from build123d import *

# Parameters (mm, degrees)
F0_W     = 38
F0_H     = 38
F0_R     = 2.25
F0_R_2   = 3.5
F1_DEPTH = 4
F2_DEPTH = 1
F3_DEPTH = 6
F4_R     = 5


with BuildPart() as f1:
    # F0 (on Top) → F1 (new body)
    with BuildSketch(Plane.XY):
        Rectangle(F0_W, F0_H)
        with Locations((-13, -13)):
            Circle(F0_R, mode=Mode.SUBTRACT)
        with Locations((13, -13)):
            Circle(F0_R, mode=Mode.SUBTRACT)
        with Locations((-13, 13)):
            Circle(F0_R, mode=Mode.SUBTRACT)
        Circle(F0_R_2, mode=Mode.SUBTRACT)
        with Locations((13, 13)):
            Circle(F0_R, mode=Mode.SUBTRACT)
        Circle(F0_R_2)
        Circle(F0_R, mode=Mode.SUBTRACT)
        Circle(F0_R)
    extrude(amount=-F1_DEPTH)

    # F0 (on Top) → F2 (join)
    with BuildSketch(Plane.XY):
        Circle(F0_R_2)
        Circle(F0_R, mode=Mode.SUBTRACT)
    extrude(amount=F2_DEPTH)

    # F0 (on Top) → F3 (join)
    with BuildSketch(Plane.XY):
        Circle(F0_R)
    extrude(amount=F3_DEPTH)

    # F4
    f4_edges = [f1.edges().sort_by_distance(p)[0] for p in [
        (-19, -19, -2),
        (19, -19, -2),
        (19, 19, -2),
        (-19, 19, -2),
    ]]
    fillet(f4_edges, radius=F4_R)


solid = f1.part
Input: part model. Units: mm. Frame: model coordinates. A direction names the side the tool comes from. Coordinates: 2 decimals unless noted, no trailing zeros. Order: outer loops, then holes, each group sorted by start corner. A loop starts at its lowest first (then second) coordinate and runs counter-clockwise, first axis right, second up.
1. Cut plane D-D, the plane y = 0. Return loops of the section in (x, z).
Checked values:
outline: (-19, -4) - (19, -4) - (19, 0) - (3.5, 0) - (3.5, 1) - (2.25, 1) - (2.25, 6) - (-2.25, 6) - (-2.25, 1) - (-3.5, 1) - (-3.5, 0) - (-19, 0) - close
2. Ray query, line 1 along Y through (x, z) = (13, -1.7); line 2 along Z through (x, y) = (8.5, 16.5); line 3 along X through (y, z) = (2, 3.5). Return the intervals inside material, ascending.
Checked values:
line 1: y = -19 to -15.25, -10.75 to 10.75, 15.25 to 19
line 2: z = -4 to 0
line 3: x = -1.03 to 1.03
3. Access query for faces 1 (the flat face through (0.7, -2.3, 1)), 2 (the flat face through (0, -19, -2)). Directions: +Z, -Z, +X, -X, +Y, -Y. A direction counts if a zero-diameter tool reaches every point of the face in a straight line with its end or side. Return the directions, or none.
Checked values:
face 1: +Z
face 2: +Z, -Z, +X, -X, -Y
4. Cut plane C-C, the plane z = -3.25. Return loops of the section in (x, y), plus the area to 3 significant figures.
Checked values:
outline: (-19, -14) arc R5 ccw to (-14, -19) - (14, -19) arc R5 ccw to (19, -14) - (19, 14) arc R5 ccw to (14, 19) - (-14, 19) arc R5 ccw to (-19, 14) - close; hole circle Ø4.5 at (-13, -13); hole circle Ø4.5 at (-13, 13); hole circle Ø4.5 at (13, -13); hole circle Ø4.5 at (13, 13)
area: 1,360 mm2
5. Draft query along X for faces 3 (the cylindrical face through (17, -18, -2)), 4 (the flat face through (-4, 0, 0)), 5 (the cylindrical face through (-14.66, 14.52, -1.97)). Return one class per face: +X half, -X half, draft (parallel to the pull), parting line (faces both ways), or undercut.
Checked values:
face 3: +X half
face 4: draft
face 5: undercut
6. Cut plane A-A, the plane y = 13. Return loops of the section in (x, z), plus the area to 3 significant figures.
Checked values:
outline: (-19, -4) - (-15.25, -4) - (-15.25, 0) - (-19, 0) - close; (-10.75, -4) - (10.75, -4) - (10.75, 0) - (-10.75, 0) - close; (15.25, -4) - (19, -4) - (19, 0) - (15.25, 0) - close
area: 116 mm2
7. Contact query for flat-ended pins moving along their axis: P1, Ø6, axis at x = -13, y = -13, coming from the +Z side; P2, Ø1, axis at y = 15, z = -1, coming from the +X side; P3, Ø19, axis at x = 5.5, y = 1, coming from the +Z side; P4, Ø3.5, axis at x = -13, y = 13, coming from the +Z side. Output: stop coordinate, or through.
Checked values:
P1: stops at z = 0
P2: stops at x = 18.97
P3: stops at z = 6
P4: passes through
